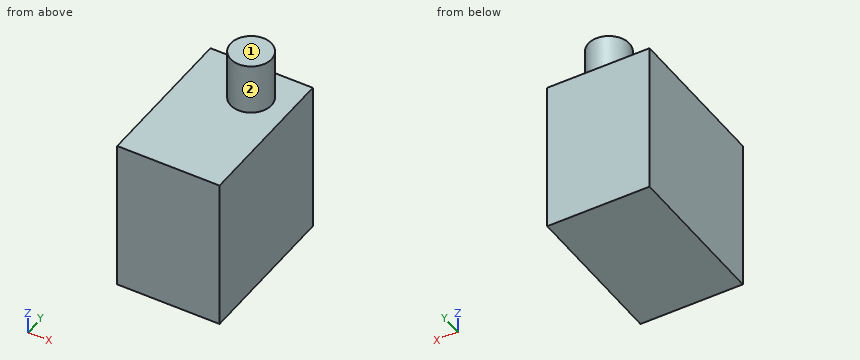
from build123d import *

# Parameters (mm, degrees)
SKETCH002_R  = 4
PAD001_DEPTH = 10
SKETCH_W     = 30
SKETCH_H     = 30
PAD_DEPTH    = 20


with BuildPart() as pad001:
    # Sketch002 → Pad001 (new body)
    with BuildSketch(Plane.XY.offset(-10)):
        Circle(SKETCH002_R)
    extrude(amount=PAD001_DEPTH)


with BuildPart() as fusion004:
    # Sketch → Pad (new body)
    with BuildSketch(Plane.YZ.offset(7.5)):
        with Locations((-7.5, -25)):
            Rectangle(SKETCH_W, SKETCH_H)
    extrude(amount=-PAD_DEPTH)

    # Fusion004: union Pad001
    add(pad001.part)


solid = fusion004.part
Design review of the part built by this model. Coordinates are the model's own, in mm. Face numbers are marked on the shaded views. A direction names the side the tool comes from. Give positions to 0.01 mm unless a question says otherwise; leave off trailing zeros. Write each loop counter-clockwise with the first axis right and the second up, starting at its lowest first coordinate (ties: lowest second). Pieces come first, ordered by that corner, then holes. Notation, with made-up numbers: M -22.5,23 L 19.5,23 A13 cw 19.5,45 Z; hole C -39,-26 d3. An arc over 180 degrees is marked long. Answer as a JSON object with one key per item and string values. Group by question number.
1) Tool access review of the marked faces 1 and 2: name each direction out of +Z, -Z, +X, -X, +Y, -Y from which nothing blocks a thin tool from reaching the whole face with its end or side.
2) We need section D-D (x = -10.5). Give the boundary of the cut face in (y, z).
3) We need section B-B (y = 0). Give the boundary of the cut face in (x, z).
4) For line 1 along Z through (x, y) = (-8, -18); line 2 along X through (y, z) = (1.75, -6); line 3 along X through (y, z) = (-3.25, -8), list the stretches that pass through material, from the lowest coordinate up.
5) We need section A-A (x = 0). Give the boundary of the cut face in (y, z), and give its area (3 significant figures).
6) Clearance check with flat-ended pins moving along their axes: pin 1 Ø1 at (x, z) = (0.5, -6.5) entering from +Y; pin 2 Ø6 at (x, y) = (2.5, -7) entering from +Z; pin 3 Ø2 at (y, z) = (1.5, -7.5) entering from +X. State where each tip first meets the part, or that it passes through.
7) We need section C-C (z = -7.5). Give the boundary of the cut face in (x, y).
Answer key:
{
 "1": {"face 1": "+Z, +X, -X, +Y, -Y", "face 2": "+Z"},
 "2": {"outline": "M -22.5,-40 L 7.5,-40 L 7.5,-10 L -22.5,-10 Z"},
 "3": {"outline": "M -12.5,-40 L 7.5,-40 L 7.5,-10 L 4,-10 L 4,0 L -4,0 L -4,-10 L -12.5,-10 Z"},
 "4": {"line 1": "z = -40 to -10", "line 2": "x = -3.6 to 3.6", "line 3": "x = -2.33 to 2.33"},
 "5": {"outline": "M -22.5,-40 L 7.5,-40 L 7.5,-10 L 4,-10 L 4,0 L -4,0 L -4,-10 L -22.5,-10 Z", "area": "980 mm²"},
 "6": {"pin 1": "stops at y = 4", "pin 2": "stops at z = -10", "pin 3": "stops at x = 3.97"},
 "7": {"outline": "C 0,0 d8"}
}
